Autodesk Inventor part; units mm, degrees
ref_plane "YZ Plane" through (0, 0, 0) normal (1, 0, 0) x (0, 1, 0)
ref_plane "XZ Plane" through (0, 0, 0) normal (0, 1, 0) x (-1, 0, 0)
ref_plane "XY Plane" through (0, 0, 0) normal (0, 0, 1) x (1, 0, 0)
sketch "Sketch8" plane through (0, 0, 0) normal (0, 1, 0) x (-1, 0, 0)
  circle A0 centre (0, 0) radius 4.25
  line L0 (-1.5588, -2.7) -> (-3.1177, 0)
  line L1 (-3.1177, 0) -> (-1.5588, 2.7)
  line L2 (-1.5588, 2.7) -> (1.5588, 2.7)
  line L3 (1.5588, 2.7) -> (3.1177, 0)
  line L4 (3.1177, 0) -> (1.5588, -2.7)
  line L5 (1.5588, -2.7) -> (-1.5588, -2.7)
  line L6 (-5.95, 0) -> (5.95, 0)
  dimension "d57" = 8.5
  dimension "d58" = 5.4
extrude "Extrusion7" add sketch "Sketch8" along normal blind 4 contours L6 L3 L2 L1 A0 | A0 L6 L0 L5 L4
sketch "Sketch9" plane through (0, 4, 0) normal (0, 1, 0) x (1, 0, 0)
  circle A0 centre (0, 0) radius 4.25
  line L0 (-3.1177, 0) -> (-1.5588, 2.7)
  line L1 (-1.5588, 2.7) -> (1.5588, 2.7)
  line L2 (1.5588, 2.7) -> (3.1177, 0)
  line L3 (3.1177, 0) -> (1.5588, -2.7)
  line L4 (1.5588, -2.7) -> (-1.5588, -2.7)
  line L5 (-1.5588, -2.7) -> (-3.1177, 0)
  circle A1 centre (0, 0) radius 2.55
  dimension "d61" = 5.1
extrude "Extrusion8" add sketch "Sketch9" along normal blind 30 contours A0 | L0 L1 L2 L3 L4 L5
properties part number "30_Cube_Z_Focus_MGN_NEMA_Motorcoupling_Captive_v3"
Build history of the part. All positions in model axes, mm. A direction names the side the tool comes from. Round coordinates to 2 decimals unless told otherwise and drop trailing zeros. Loops run counter-clockwise (first coordinate to the right, second up) from the corner with the lowest first, then second, coordinate; pieces in that order, holes last. Notation, with made-up numbers: (-38.5, 26) -> (-20.5, 26) arc R18 cw to (-20.5, 39) -> close; hole circle Ø8 at (72.5, 47.5). An arc over 180 degrees is marked (long way). One line per item, written item: value. Start each with the question number.
Q1. Cut at A-A on y = 13. List the corners of the cut face in (x, z).
Q2. Probe line 1 along Z through (x, y) = (0, 12); line 2 along Z through (x, y) = (1, 3.5). List the from-to ranges inside material, lowest first.
Q3. Drop flat-ended pins along their axis: pin 1 Ø1 at (y, z) = (8.5, 3) entering from -X; pin 2 Ø1 at (x, y) = (-2.5, 21.5) entering from -Z; pin 3 Ø1.6 at (x, z) = (-0.5, -0.5) entering from -Y. Give the stop position or say it passes through.
Q4. Two-plate mould, pull along Z, no slides. Class faces 1 (the face through (0.28, 16.76, 4.24)), 2 (the face through (0, 0, -3)), 3 (the face through (0, 2, 2.7)): released by +Z, released by -Z, zero draft, split by the parting line, or undercut.
Q5. 3-axis set-ups, long thin cutter, end or side, ignore diameter. For faces 4 (the face through (2, 34, 2)), 5 (the face through (-2.327, 1.972, 1.369)): which of +Z, -Z, +X, -X, +Y, -Y reach the whole face in a straight line?
Q6. Cut at C-C on z = -3. List the corners of the cut face in (x, y).
Computed:
1. outline: circle Ø8.5 at (0, 0); hole circle Ø5.1 at (0, 0)
2. line 1: -4.25 to -2.55, 2.55 to 4.25
2. line 2: -4.13 to -2.7, 2.7 to 4.13
3. pin 1: x = -3.44
3. pin 2: z = -3.75
3. pin 3: through
4. face 1: split by the parting line
4. face 2: zero draft
4. face 3: undercut
5. face 4: +Z, -Z, +X, -X, +Y
5. face 5: -Y
6. outline: (-3.01, 0) -> (3.01, 0) -> (3.01, 34) -> (-3.01, 34) -> close
